Check sheet for the drawn part. Datum: minimum x, y, z corner. Units: mm. Give positions to 0.01 mm unless a question says otherwise; leave off trailing zeros. Write each loop counter-clockwise with the first axis right and the second up, starting at its lowest first coordinate (ties: lowest second). Pieces come first, ordered by that corner, then holes. Notation, with made-up numbers: (5.5, 12.5) - (26.5, 12.5) arc R25 cw to (26.5, 42.5) - close; hole circle Ø3 at (-4.75, 35.25). An arc over 180 degrees is marked (long way). Return JSON: item names as keys, results as strings. Group by question number.
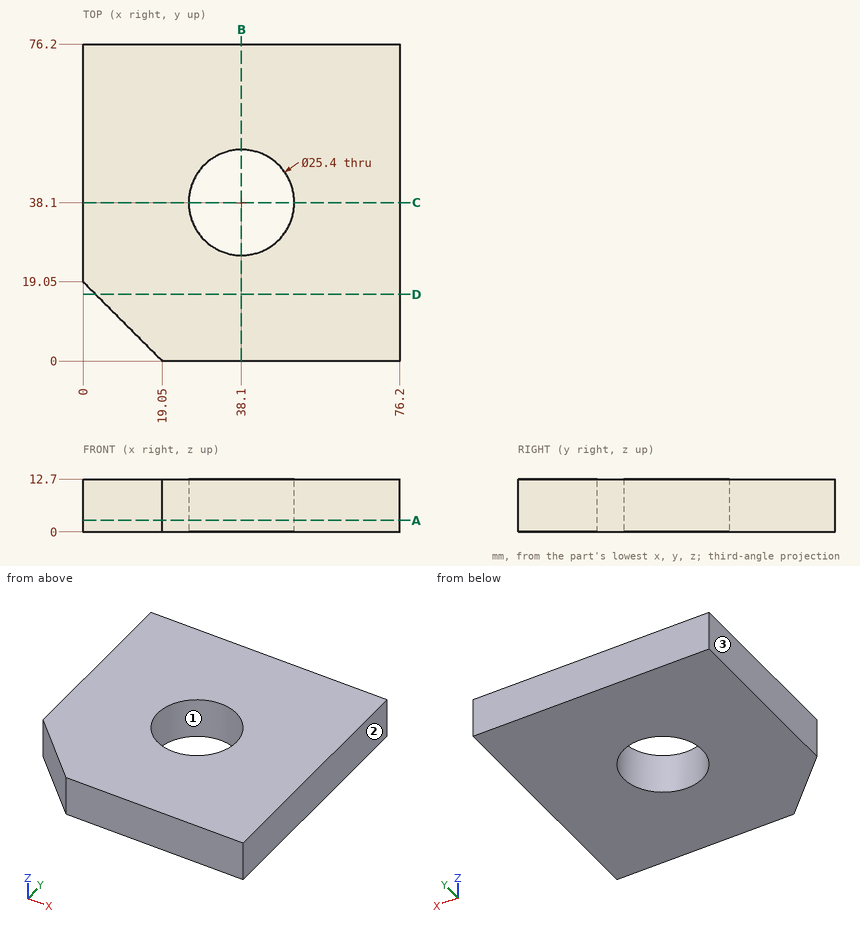
Item 1: Material ranges on line 1 along Y through (x, z) = (38.1, 5.75); line 2 along Y through (x, z) = (33, 3.5); line 3 along X through (y, z) = (11.5, 9.75), recorded low to high. Write a range as from..to.
Item 2: Section check A-A on z = 2.75. Record the cut outline in (x, y), plus the area to 3 significant figures.
Item 3: Mould release check, pull along X, two halves, no side actions. Record for the marked faces 1, 2 and 3: +X half, -X half, draft (parallel to the pull), parting line (faces both ways), or undercut.
Item 4: Section check B-B on x = 38.1. Record the cut outline in (y, z).
Item 5: Section check D-D on y = 16. Record the cut outline in (x, z), plus the area to 3 significant figures.
Reply:
{
 "1": {"line 1": "0..25.4, 50.8..76.2", "line 2": "0..26.47, 49.73..76.2", "line 3": "7.55..76.2"},
 "2": {"outline": "(0, 19.05) - (19.05, 0) - (76.2, 0) - (76.2, 76.2) - (0, 76.2) - close; hole circle Ø25.4 at (38.1, 38.1)", "area": "5,120 mm²"},
 "3": {"face 1": "undercut", "face 2": "+X half", "face 3": "-X half"},
 "4": {"outline": "(0, 0) - (25.4, 0) - (25.4, 12.7) - (0, 12.7) - close; (50.8, 0) - (76.2, 0) - (76.2, 12.7) - (50.8, 12.7) - close"},
 "5": {"outline": "(3.05, 0) - (76.2, 0) - (76.2, 12.7) - (3.05, 12.7) - close", "area": "929 mm²"}
}
